Part model, mm, in its own coordinate system. Face numbers are marked on the shaded views. A direction names the side the tool comes from. Round coordinates to 2 decimals unless told otherwise and drop trailing zeros. Loops run counter-clockwise (first coordinate to the right, second up) from the corner with the lowest first, then second, coordinate; pieces in that order, holes last.
from build123d import *

# Parameters (mm, degrees)
SKETCH1_W           = 109.1
SKETCH1_H           = 40
BOSS_EXTRUDE1_DEPTH = 8
SKETCH2_W           = 22.3
SKETCH2_H           = 48
BOSS_EXTRUDE2_DEPTH = 8
SKETCH3_W           = 49.3
SKETCH3_H           = 60
BOSS_EXTRUDE3_DEPTH = 8
SKETCH4_W           = 49.3
SKETCH4_H           = 60
BOSS_EXTRUDE4_DEPTH = 6
SKETCH5_R           = 3.25
CUT_EXTRUDE1_DEPTH  = 11.1
SKETCH6_R           = 3.25
CUT_EXTRUDE2_DEPTH  = 11.1
SKETCH7_R           = 2.05
CUT_EXTRUDE3_DEPTH  = 6.7
SKETCH8_W           = 26
SKETCH8_H           = 12
BOSS_EXTRUDE5_DEPTH = 3.25
SKETCH9_W           = 26
SKETCH9_H           = 12
BOSS_EXTRUDE6_DEPTH = 3


with BuildPart() as part:
    # Sketch1 → Boss-Extrude1 (new body)
    with BuildSketch(Plane.XY.offset(246)):
        with Locations((281.75, 300)):
            Rectangle(SKETCH1_W, SKETCH1_H)
        with BuildLine():
            Line((290, 296), (290, 304))
            ThreePointArc((290, 304), (288, 306), (286, 304))
            Line((286, 304), (286, 296))
            ThreePointArc((286, 296), (288, 294), (290, 296))
        make_face(mode=Mode.SUBTRACT)
        with BuildLine():
            Line((304, 296), (304, 304))
            ThreePointArc((304, 304), (302, 306), (300, 304))
            Line((300, 304), (300, 296))
            ThreePointArc((300, 296), (302, 294), (304, 296))
        make_face(mode=Mode.SUBTRACT)
    extrude(amount=BOSS_EXTRUDE1_DEPTH)

    # Sketch2 → Boss-Extrude2 (add)
    with BuildSketch(Plane.XY.offset(246)):
        with Locations((325.15, 300)):
            Rectangle(SKETCH2_W, SKETCH2_H)
    extrude(amount=BOSS_EXTRUDE2_DEPTH)

    # Sketch3 → Boss-Extrude3 (add)
    with BuildSketch(Plane.XY.offset(246)):
        with Locations((251.85, 300)):
            Rectangle(SKETCH3_W, SKETCH3_H)
    extrude(amount=BOSS_EXTRUDE3_DEPTH)

    # Sketch4 → Boss-Extrude4 (add)
    with BuildSketch(Plane.XY.offset(254)):
        with Locations((251.85, 300)):
            Rectangle(SKETCH4_W, SKETCH4_H)
    extrude(amount=BOSS_EXTRUDE4_DEPTH)

    # Sketch5 → Cut-Extrude1 (cut)
    with BuildSketch(Plane.XY.offset(248.9)):
        with Locations((238, 290.5)):
            Circle(SKETCH5_R)
        with Locations((238, 309.5)):
            Circle(SKETCH5_R)
    extrude(amount=CUT_EXTRUDE1_DEPTH, mode=Mode.SUBTRACT)

    # Sketch6 → Cut-Extrude2 (cut)
    with BuildSketch(Plane.XY.offset(246)):
        with Locations((252, 281)):
            Circle(SKETCH6_R)
        with Locations((252, 319)):
            Circle(SKETCH6_R)
        with Locations((266, 281)):
            Circle(SKETCH6_R)
        with Locations((266, 319)):
            Circle(SKETCH6_R)
    extrude(amount=CUT_EXTRUDE2_DEPTH, mode=Mode.SUBTRACT)

    # Sketch7 → Cut-Extrude3 (cut)
    with BuildSketch(Plane.XY.offset(247.3)):
        with Locations(Location((320, 282.7, 0), (0, 0, 180))):
            Circle(SKETCH7_R)
        with Locations(Location((320, 317.3, 0), (0, 0, 180))):
            Circle(SKETCH7_R)
        with Locations(Location((329.5, 282.7, 0), (0, 0, 180))):
            Circle(SKETCH7_R)
        with Locations(Location((329.5, 317.3, 0), (0, 0, 180))):
            Circle(SKETCH7_R)
    extrude(amount=CUT_EXTRUDE3_DEPTH, mode=Mode.SUBTRACT)

    # Sketch8 → Boss-Extrude5 (add)
    with BuildSketch(Plane.XY.offset(254)):
        with Locations((293, 298)):
            Rectangle(SKETCH8_W, SKETCH8_H)
    extrude(amount=BOSS_EXTRUDE5_DEPTH)

    # Sketch9 → Boss-Extrude6 (add)
    with BuildSketch(Plane.XY.offset(254)):
        with Locations((293, 302)):
            Rectangle(SKETCH9_W, SKETCH9_H)
    extrude(amount=BOSS_EXTRUDE6_DEPTH)


solid = part.part
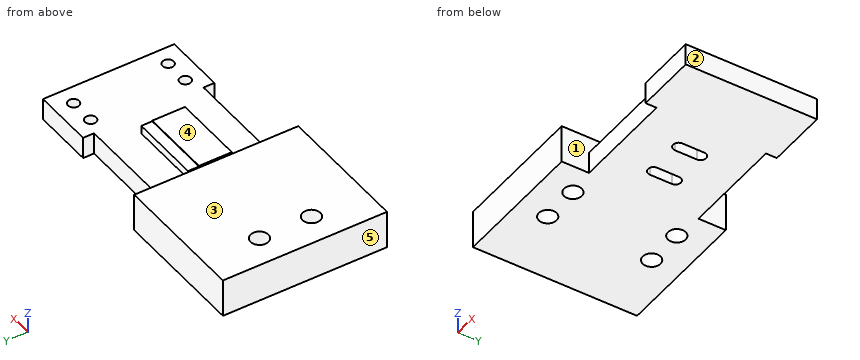
1) Slice it at B-B, the plane y = 300. Give the cut face in (x, z), then the cut area to 3 significant figures.
Values:
outline: (227.2, 246) - (286, 246) - (286, 254) - (290, 254) - (290, 246) - (300, 246) - (300, 254) - (304, 254) - (304, 246) - (336.3, 246) - (336.3, 254) - (306, 254) - (306, 257.25) - (280, 257.25) - (280, 254) - (276.5, 254) - (276.5, 260) - (227.2, 260) - close
area: 1,190 mm2
2) Slice it at A-A, the plane z = 252. Give the number of separate pieces and of enclosed holes in the cut face, then the cut area to 3 significant figures.
Values:
separate pieces: 1
enclosed holes: 12
area: 5,190 mm2
3) Drop flat-ended pins along their axis: pin 1 Ø6 at (x, z) = (300, 255) entering from -Y; pin 2 Ø6 at (y, z) = (295.5, 256) entering from +X; pin 3 Ø9.5 at (x, y) = (287, 298) entering from +Z; pin 4 Ø2 at (x, y) = (319.5, 318) entering from +Z. Give the stop position or say it passes through.
Values:
pin 1: stops at y = 280
pin 2: stops at x = 336.3
pin 3: stops at z = 257.25
pin 4: stops at z = 247.3
4) Wall check: line 1 along Y through (x, z) = (320, 251); line 2 along Y through (x, z) = (252, 253); line 3 along X through (y, z) = (290.5, 256.25). Give the ranges that are in metal, low to high.
Values:
line 1: y = 276 to 280.65, 284.75 to 315.25, 319.35 to 324
line 2: y = 270 to 277.75, 284.25 to 315.75, 322.25 to 330
line 3: x = 227.2 to 234.75, 241.25 to 276.5
5) Mould opens along X. For the marked faces 1, 2 and 3 say: released by +X, released by -X, zero draft, split by the parting line, or undercut.
Values:
face 1: undercut
face 2: released by +X
face 3: zero draft
6) Slice it at C-C, the plane x = 266. Give the cut face in (y, z).
Values:
outline: (270, 246) - (277.75, 246) - (277.75, 257.1) - (284.25, 257.1) - (284.25, 246) - (315.75, 246) - (315.75, 257.1) - (322.25, 257.1) - (322.25, 246) - (330, 246) - (330, 260) - (270, 260) - close
7) Slice it at D-D, the plane y = 290.5. Give the cut face in (x, z), then the cut area to 3 significant figures.
Values:
outline: (227.2, 246) - (336.3, 246) - (336.3, 254) - (276.5, 254) - (276.5, 260) - (241.25, 260) - (241.25, 248.9) - (234.75, 248.9) - (234.75, 260) - (227.2, 260) - close
area: 1,100 mm2
8) Tool access for the marked faces 4 and 5: list every direction of +Z, -Z, +X, -X, +Y, -Y with a clear straight run to the whole face (end or side of a thin tool).
Values:
face 4: +Z, +X, +Y, -Y
face 5: +Z, -Z, -X, +Y, -Y
